Check sheet for the modelled part. Datum: model origin and axes. Units: mm. Give positions to 0.01 mm unless a question says otherwise; leave off trailing zeros. Order: outer loops, then holes, each group sorted by start corner. A loop starts at its lowest first (then second) coordinate and runs counter-clockwise, first axis right, second up. Notation, with made-up numbers: (4.25, -6.5) -> (62.25, -6.5) arc R19 cw to (62.25, 2.5) -> close; hole circle Ø4 at (-7, -23.75). An arc over 180 degrees is marked (long way). Answer in a Markdown table with one row per item. Add a question column.
(1) Cross-section at B-B (x = 34.5). Record the cut outline in (y, z).
(2) Go/stop test with flat-tipped pins: pin 1 (2 mm diameter, centred on x = 9.5, z = -50.1, fed in from +Y); pin 2 (3 mm diameter, centred on x = 40, z = -76, fed in from +Y); pin 3 (5 mm diameter, centred on x = 7, z = -59, fed in from +Y) (3 decimals). Record where each tip stops, or that it passes through.
(3) Thickness scan on L1, parallel to X at y = 2.55, z = -22.5; L2, parallel to X at y = 3.05, z = -58; L3, parallel to X at y = 3.45, z = -59. Record the ranges inside material, lowest first. Write a range as [from, to].
(4) Cross-section at C-C (z = -20). Record the cut outline in (x, y).
(5) Cross-section at A-A (z = -63). Record the cut outline in (x, y).
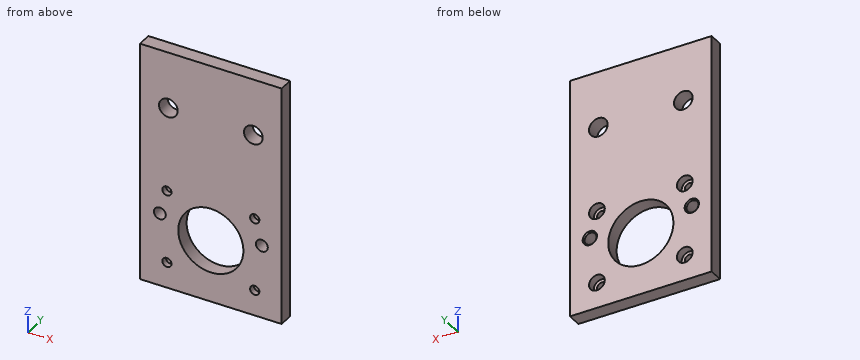
```python
from build123d import *

# Parameters (mm, degrees)
SKETCH1_W                                      = 50
SKETCH1_H                                      = 85
SKETCH1_R                                      = 11.5
BOSS_EXTRUDE1_DEPTH                            = 5
CBORE_FOR_4_SOCKET_HEAD_CAP_SCREW1_D           = 3.2639
CBORE_FOR_4_SOCKET_HEAD_CAP_SCREW1_CBORE_D     = 5.55752
CBORE_FOR_4_SOCKET_HEAD_CAP_SCREW1_CBORE_DEPTH = 2.8448
M6_CLEARANCE_HOLE1_D                           = 6.6
M5_TAPPED_HOLE1_D                              = 4.2
M5_TAPPED_HOLE1_CSINK_D                        = 5.05
M5_TAPPED_HOLE1_CSINK_ANGLE                    = 90


with BuildPart() as part:
    # Sketch1 → Boss-Extrude1 (new body)
    with BuildSketch(Plane(origin=(0, 0, 0), x_dir=(1, 0, 0), z_dir=(0, 1, 0))):
        with Locations((25, 42.5)):
            Rectangle(SKETCH1_W, SKETCH1_H)
        with Locations(Location((25, 63, 0), (0, 0, 270))):
            Circle(SKETCH1_R, mode=Mode.SUBTRACT)
    extrude(amount=BOSS_EXTRUDE1_DEPTH)

    # CBORE for #4 Socket Head Cap Screw1 (through all)
    with Locations(Plane(origin=(0, 5, 0), x_dir=(-1, 0, 0), z_dir=(0, 1, 0))):
        with Locations((-9.5, -75.903324015), (-9.5, -50.096675985), (-40.5, -50.096675985), (-40.5, -75.903324015)):
            CounterBoreHole(CBORE_FOR_4_SOCKET_HEAD_CAP_SCREW1_D / 2, CBORE_FOR_4_SOCKET_HEAD_CAP_SCREW1_CBORE_D / 2, CBORE_FOR_4_SOCKET_HEAD_CAP_SCREW1_CBORE_DEPTH)

    # M6 Clearance Hole1 (through all)
    with Locations(Plane(origin=(0, 5, 0), x_dir=(-1, 0, 0), z_dir=(0, 1, 0))):
        with Locations((-10, -20), (-40, -20)):
            Hole(M6_CLEARANCE_HOLE1_D / 2)

    # M5 Tapped Hole1 (through all)
    with Locations(Plane(origin=(0, 5, 0), x_dir=(-1, 0, 0), z_dir=(0, 1, 0))):
        with Locations((-7, -59), (-43, -59)):
            CounterSinkHole(M5_TAPPED_HOLE1_D / 2, M5_TAPPED_HOLE1_CSINK_D / 2, counter_sink_angle=M5_TAPPED_HOLE1_CSINK_ANGLE)


solid = part.part
```
Answer below:
| question | item | result |
|---|---|---|
| 1 | outline | (0, -85) -> (5, -85) -> (5, -69.48) -> (0, -69.48) -> close; (0, -56.52) -> (5, -56.52) -> (5, 0) -> (0, 0) -> close |
| 2 | pin 1 | passes through |
| 2 | pin 2 | stops at y = 2.16 |
| 2 | pin 3 | stops at y = 4.975 |
| 3 | L1 | x = [0, 7.85], [12.15, 37.85], [42.15, 50] |
| 3 | L2 | x = [0, 5.15], [8.85, 14.64], [35.36, 41.15], [44.85, 50] |
| 3 | L3 | x = [0, 4.9], [9.1, 14.22], [35.78, 40.9], [45.1, 50] |
| 4 | outline | (0, 0) -> (6.7, 0) -> (6.7, 5) -> (0, 5) -> close; (13.3, 0) -> (36.7, 0) -> (36.7, 5) -> (13.3, 5) -> close; (43.3, 0) -> (50, 0) -> (50, 5) -> (43.3, 5) -> close |
| 5 | outline | (0, 0) -> (13.5, 0) -> (13.5, 5) -> (0, 5) -> close; (36.5, 0) -> (50, 0) -> (50, 5) -> (36.5, 5) -> close |
